```python
from build123d import *

# Parameters (mm, degrees)
F0_W     = 18
F0_H     = 8
F1_DEPTH = 3
F2_W     = 16
F2_H     = 8
F3_DEPTH = 60
F4_R     = 0.99999
F5_W     = 24
F5_H     = 8
F6_DEPTH = 35
F7_R     = 3
F8_R     = 4
F9_DEPTH = 2


# Not quite as in the source:
# - a fillet or chamfer is up to 0.001 mm smaller than in the source, because OpenCascade refuses the exact size


with BuildPart() as f1:
    # F0 (on Front) → F1 (new body)
    with BuildSketch(Plane.XZ):
        Rectangle(F0_W, F0_H)
    extrude(amount=F1_DEPTH)

    # F2 (on face) → F3 (join)
    with BuildSketch(Plane.XZ.offset(3)):
        Rectangle(F2_W, F2_H)
    extrude(amount=F3_DEPTH)

    # F4 (radius 1 in the source; OpenCascade refuses exactly that, so slightly less here)
    f4_edges = [f1.edges().sort_by_distance(p)[0] for p in [
        (-8, -3, 0),
        (8, -3, 0),
    ]]
    fillet(f4_edges, radius=F4_R)

    # F5 (on face) → F6 (join)
    with BuildSketch(Plane.XZ.offset(63)):
        Rectangle(F5_W, F5_H)
    extrude(amount=F6_DEPTH)

    # F7
    f7_edges = [f1.edges().sort_by_distance(p)[0] for p in [
        (-12, -63, 0),
        (-12, -98, 0),
        (12, -98, 0),
        (12, -63, 0),
    ]]
    fillet(f7_edges, radius=F7_R)

    # F8 (on face) → F9 (cut)
    with BuildSketch(Plane.XY.offset(4)):
        with Locations((-5, -75)):
            Circle(F8_R)
        with Locations((3, -88)):
            Circle(F8_R)
    extrude(amount=-F9_DEPTH, mode=Mode.SUBTRACT)


solid = f1.part
```
Could you check a few things on this model? Use its own coordinates, in mm. A direction names the side the tool comes from. Coordinates: 2 decimals unless noted, no trailing zeros. Write each loop counter-clockwise with the first axis right and the second up, starting at its lowest first coordinate (ties: lowest second). Pieces come first, ordered by that corner, then holes. Notation, with made-up numbers: (-17.5, 55) -> (-10.5, 55) arc R14 ccw to (-10.5, 70) -> close; hole circle Ø5 at (17, -26). An arc over 180 degrees is marked (long way). Write item = value, one per line. Start each with the question number.
(1) I want a section at B-B (x = 3). Please give me the cut outline in (y, z), plus the area to 3 significant figures.
(2) I want a section at C-C (y = -75). Please give me the cut outline in (x, z), plus the area to 3 significant figures.
(3) I want a section at D-D (y = -16). Please give me the cut outline in (x, z), plus the area to 3 significant figures.
(4) Which directions (+Z, -Z, +X, -X, +Y, -Y) give clear straight access to the entire face, cutting with the end or side of a thin tool? Please do faces 1 (the face through (-8, -33, 0)), 2 (the face through (3, -88, 2)), 3 (the face through (9, -1, 0)), 4 (the face through (8, -33, 0)), 5 (the face through (-9, -1, 0)).
(5) Will these pins go through, and if not, where does the flat tip stop? pin 1 (0.9 mm diameter, centred on y = -2, z = 0, fed in from -X); pin 2 (1.5 mm diameter, centred on x = -5.5, y = -74.5, fed in from +Z); pin 3 (1.5 mm diameter, centred on y = -32.5, z = -1, fed in from -X).
(6) I need wall thicknesses on line 1 (Y direction, x = 3, z = 2.55); line 2 (Y direction, x = -5, z = 3.5); line 3 (Y direction, x = 9.25, z = 1.25). Which ranges of each line are inside material? Lowest first, please. Write a range as [from, to].
(7) We'd pull the mould along Y, two halves only. Please class faces 6 (the face through (-5, -75, 2)), 7 (the face through (0, -48, -4)), 8 (the face through (-11.14, -97.1, 0.06)): released by +Y, released by -Y, zero draft, split by the parting line, or undercut.
Result set:
q1.outline = (-98, -4) -> (0, -4) -> (0, 4) -> (-84, 4) -> (-84, 2) -> (-92, 2) -> (-92, 4) -> (-98, 4) -> close
q1.area = 768 mm2
q2.outline = (-12, -4) -> (12, -4) -> (12, 4) -> (-1, 4) -> (-1, 2) -> (-9, 2) -> (-9, 4) -> (-12, 4) -> close
q2.area = 176 mm2
q3.outline = (-8, -4) -> (8, -4) -> (8, 4) -> (-8, 4) -> close
q3.area = 128 mm2
q4.face_1 = +Z, -Z, -X
q4.face_2 = +Z
q4.face_3 = +Z, -Z, +X, +Y
q4.face_4 = +Z, -Z, +X
q4.face_5 = +Z, -Z, -X, +Y
q5.pin_1 = -9
q5.pin_2 = 2
q5.pin_3 = -8
q6.line_1 = [-98, -92], [-84, 0]
q6.line_2 = [-98, -79], [-71, 0]
q6.line_3 = [-97.99, -63.01]
q7.face_6 = undercut
q7.face_7 = zero draft
q7.face_8 = released by -Y
